```python
from build123d import *

# Parameters (mm, degrees)
SKETCH1_R           = 2.25
BOSS_EXTRUDE1_DEPTH = 3


with BuildPart() as part:
    # Sketch1 → Boss-Extrude1 (new body)
    with BuildSketch(Plane(origin=(0, 0, 0), x_dir=(1, 0, 0), z_dir=(0, 1, 0))):
        Polygon((-15, 10), (-15, 5), (-18, 5), (-18, -5), (-15, -5), (-15, -10), (15, -10), (15, -5), (18, -5), (18, 5), (15, 5), (15, 10), align=None)
        Circle(SKETCH1_R, mode=Mode.SUBTRACT)
    extrude(amount=BOSS_EXTRUDE1_DEPTH)


solid = part.part
```
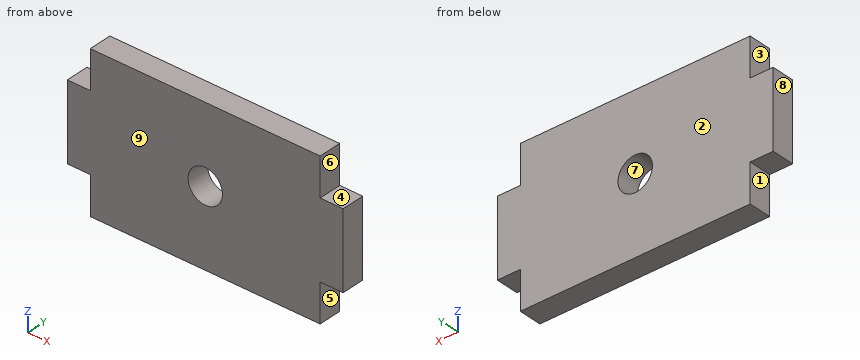
Geometry check sheet. Reference: the model listing, model coordinates, mm. Face numbers are marked on the shaded views. A direction names the side the tool comes from. Round coordinates to 2 decimals unless told otherwise and drop trailing zeros. Loops run counter-clockwise (first coordinate to the right, second up) from the corner with the lowest first, then second, coordinate; pieces in that order, holes last. Notation, with made-up numbers: (48.25, 84) - (96.25, 84) arc R21 ccw to (96.25, 108) - close; hole circle Ø7 at (4, -40). An arc over 180 degrees is marked (long way). Write item = value, one per line. Start each with the question number.
1. Section check B-B on x = 0. Enter the section's corners in (y, z), then the cut area to 3 significant figures.
2. Set-up check for the marked faces 1, 2, 3, 4 and 5: record each of +Z, -Z, +X, -X, +Y, -Y from which the full face is reachable in a straight line by a thin tool's end or side.
3. Depth check by flat-ended pin: pin 1 (0.9 mm diameter, centred on x = 17, y = 1, fed in from -Z); pin 2 (0.9 mm diameter, centred on y = 2, z = -8, fed in from -X); pin 3 (1.5 mm diameter, centred on x = 17, y = 1.5, fed in from +Z). Enter the tip coordinate at first touch or a pass-through.
4. Section check A-A on y = 2.4. Enter the section's corners in (x, z).
5. Thickness scan on line 1 (Z direction, x = 0, y = 0.8); line 2 (X direction, y = 1, z = 0); line 3 (Z direction, x = 16, y = 2.45). Record the ranges inside material, lowest first.
6. Section check C-C on z = 0. Enter the section's corners in (x, y), then the cut area to 3 significant figures.
7. Section check D-D on z = 7.25. Enter the section's corners in (x, y), then the cut area to 3 significant figures.
8. Mould release check, pull along X, two halves, no side actions. Record for the marked faces 6, 7, 8 and 9: released by +X, released by -X, zero draft, split by the parting line, or undercut.
Working result:
q1.outline = (0, -10) - (3, -10) - (3, -2.25) - (0, -2.25) - close; (0, 2.25) - (3, 2.25) - (3, 10) - (0, 10) - close
q1.area = 46.5 mm^2
q2.face_1 = -Z, -X, +Y, -Y
q2.face_2 = +Z, -Z, +X, -X, +Y
q2.face_3 = +Z, -X, +Y, -Y
q2.face_4 = +Z, +X, +Y, -Y
q2.face_5 = -Z, +X, +Y, -Y
q3.pin_1 = -5
q3.pin_2 = -15
q3.pin_3 = 5
q4.outline = (-18, -5) - (-15, -5) - (-15, -10) - (15, -10) - (15, -5) - (18, -5) - (18, 5) - (15, 5) - (15, 10) - (-15, 10) - (-15, 5) - (-18, 5) - close; hole circle Ø4.5 at (0, 0)
q5.line_1 = -10 to -2.25, 2.25 to 10
q5.line_2 = -18 to -2.25, 2.25 to 18
q5.line_3 = -5 to 5
q6.outline = (-18, 0) - (-2.25, 0) - (-2.25, 3) - (-18, 3) - close; (2.25, 0) - (18, 0) - (18, 3) - (2.25, 3) - close
q6.area = 94.5 mm^2
q7.outline = (-15, 0) - (15, 0) - (15, 3) - (-15, 3) - close
q7.area = 90.0 mm^2
q8.face_6 = released by +X
q8.face_7 = undercut
q8.face_8 = released by -X
q8.face_9 = zero draft
